Autodesk Inventor part; units mm, degrees
ref_plane "YZ Plane" through (0, 0, 0) normal (1, 0, 0) x (0, 1, 0)
ref_plane "XZ Plane" through (0, 0, 0) normal (0, 1, 0) x (-1, 0, 0)
ref_plane "XY Plane" through (0, 0, 0) normal (0, 0, 1) x (1, 0, 0)
sketch "Sketch1" plane through (0, 0, 0) normal (0, 1, 0) x (-1, 0, 0)
  line L0 (-100, -80) -> (-100, 80)
  line L1 (100, 80) -> (100, -80)
  line L2 (100, -80) -> (-100, 80) construction
  line L3 (-100, -80) -> (100, 80) construction
  line L4 (25, -170) -> (-25, -170)
  line L5 (-25, 170) -> (25, 170)
  line L6 (25, -170) -> (-25, 170) construction
  line L7 (-25, -170) -> (25, 170) construction
  line L8 (25, 170) -> (25, 80)
  line L9 (25, -80) -> (25, -170)
  line L10 (100, -80) -> (25, -80)
  line L11 (-25, -80) -> (-100, -80)
  line L12 (-25, -170) -> (-25, -80)
  line L13 (-25, 80) -> (-25, 170)
  line L14 (-100, 80) -> (-25, 80)
  line L15 (25, 80) -> (100, 80)
  line L16 (100, 0) -> (-100, 0) construction
  line L17 (0, -170) -> (0, 170) construction
  line L18 (15, -70) -> (90, -70)
  line L19 (90, -70) -> (90, 70)
  line L20 (90, 70) -> (15, 70)
  line L21 (15, 70) -> (15, 160)
  line L22 (15, 160) -> (-15, 160)
  line L23 (-15, 160) -> (-15, 70)
  line L24 (-15, 70) -> (-90, 70)
  line L25 (-90, 70) -> (-90, -70)
  line L26 (-90, -70) -> (-15, -70)
  line L27 (-15, -70) -> (-15, -160)
  line L28 (-15, -160) -> (15, -160)
  line L29 (15, -160) -> (15, -70)
  line L30 (15, -147) -> (-15, -147)
  line L31 (15, 147) -> (-15, 147)
  point P0 (0, 0)
  dimension "d0" = 50
  dimension "d1" = 200
  dimension "d2" = 340
  dimension "d3" = 160
  dimension "d9" = 10
  dimension "d10" = 23
  dimension "d11" = 23
extrude "Extrusion1" add sketch "Sketch1" along normal mid plane 85 contours L0 L14 L13 L5 L8 L15 L1 L10 L9 L4 L12 L11 | L29 L30 L27 L26 L25 L24 L23 L31 L21 L20 L19 L18 | L29 L28 L27 L30 | L31 L23 L22 L21
chamfer "Chamfer1" distance 15 angle 45 4 edges at (0, 42.5, 170) (0, -42.5, 170) (0, 42.5, -170) (0, -42.5, -170)
extrude "Extrusion2" cut sketch "Sketch1" along normal mid plane 65 contours L29 L30 L27 L26 L25 L24 L23 L31 L21 L20 L19 L18
The model under review builds one solid part; all positions refer to its coordinate system, in mm. A direction names the side the tool comes from. Coordinates: 2 decimals unless noted, no trailing zeros. Loops run counter-clockwise (first coordinate to the right, second up) from the corner with the lowest first, then second, coordinate; pieces in that order, holes last. Notation, with made-up numbers: (21, -16.5) -> (50, -16.5) arc R31 cw to (50, 10.5) -> close; hole circle Ø10 at (76, -10.5). An arc over 180 degrees is marked (long way). Use a Markdown table: item, result. Add a question column.
1. Add section D-D on x = -20.5. Write out the cut boundary in (y, z).
2. Machinability: for faces 4 (the face through (25, 1, -126)), 5 (the face through (-15, 0, -109)), 6 (the face through (63, 1, 80)), 7 (the face through (100, 1, -1)), 8 (the face through (-62, 1, 80)), which of the approach directions +Z, -Z, +X, -X, +Y, -Y give a long, thin tool a straight path to every point of the face, cutting with its end or side? Answer none if there is none.
3. Clearance check with flat-ended pins moving along their axes: pin 1 Ø1 at (y, z) = (-11, -130) entering from +X; pin 2 Ø22.5 at (x, y) = (-77.5, -20.5) entering from +Z; pin 3 Ø3 at (x, y) = (-40.5, -31.5) entering from -Z. State where each tip first meets the part, or that it passes through.
4. Draft analysis for pull direction Y (two halves, no side actions). For faces 1 (the face through (-25, 1, 126)), 2 (the face through (-0.3, -34.9, 162.6)), 3 (the face through (-53, 0, 70)), state which applies: pulls with the +Y half, pulls with the -Y half, needs draft (parallel to the pull), parting line crosses it, or undercut.
5. To check wall thickness, follow line 1 (X direction, y = -20, z = -74.5); line 2 (Y direction, x = 38, z = -63.5); line 3 (X direction, y = -23.5, z = -6). State the ranges of each line that lie inside material, in increasing order.
6. Add section B-B on z = 114.5. Write out the cut boundary in (x, y), plus the area to 3 significant figures.
7. Add section C-C on y = -14.5. Write out the cut boundary in (x, z).
8. Add section A-A on x = -63.5. Write out the cut boundary in (y, z).
Returned:
| question | item | result |
|---|---|---|
| 1 | outline | (-42.5, -155) -> (-27.5, -170) -> (27.5, -170) -> (42.5, -155) -> (42.5, 155) -> (27.5, 170) -> (-27.5, 170) -> (-42.5, 155) -> close; hole (-32.5, -70) -> (32.5, -70) -> (32.5, 70) -> (-32.5, 70) -> close |
| 2 | face 4 | -Z, +X, +Y, -Y |
| 2 | face 5 | none |
| 2 | face 6 | +Z, +X, +Y, -Y |
| 2 | face 7 | +Z, -Z, +X, +Y, -Y |
| 2 | face 8 | +Z, -X, +Y, -Y |
| 3 | pin 1 | stops at x = 25 |
| 3 | pin 2 | stops at z = 80 |
| 3 | pin 3 | stops at z = -80 |
| 4 | face 1 | needs draft |
| 4 | face 2 | pulls with the -Y half |
| 4 | face 3 | undercut |
| 5 | line 1 | x = -100 to -15, 15 to 100 |
| 5 | line 2 | y = -42.5 to -32.5, 32.5 to 42.5 |
| 5 | line 3 | x = -100 to -90, 90 to 100 |
| 6 | outline | (-25, -42.5) -> (25, -42.5) -> (25, 42.5) -> (-25, 42.5) -> close; hole (-15, -32.5) -> (15, -32.5) -> (15, 32.5) -> (-15, 32.5) -> close |
| 6 | area | 2,300 mm² |
| 7 | outline | (-100, -80) -> (-25, -80) -> (-25, -170) -> (25, -170) -> (25, -80) -> (100, -80) -> (100, 80) -> (25, 80) -> (25, 170) -> (-25, 170) -> (-25, 80) -> (-100, 80) -> close; hole (-90, -70) -> (-15, -70) -> (-15, -147) -> (15, -147) -> (15, -70) -> (90, -70) -> (90, 70) -> (15, 70) -> (15, 147) -> (-15, 147) -> (-15, 70) -> (-90, 70) -> close |
| 8 | outline | (-42.5, -80) -> (42.5, -80) -> (42.5, 80) -> (-42.5, 80) -> close; hole (-32.5, -70) -> (32.5, -70) -> (32.5, 70) -> (-32.5, 70) -> close |
